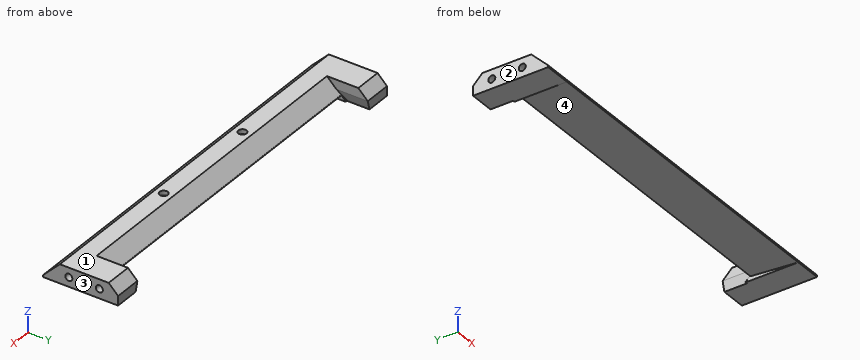
```python
from build123d import *

# Parameters (mm, degrees)
F0_W      = 520.7
F0_H      = 101.6
F1_DEPTH  = 25.4
F2_SIZE   = 22.86
F3_W      = 446.0748
F3_H      = 55.118
F4_DEPTH  = 25.401
F6_DEPTH  = 55.118
F7_SIZE   = 12.7
F9_DEPTH  = 228.6
F10_R     = 5.55625
F11_DEPTH = 6.35
F12_R     = 4.7625
F13_DEPTH = 19.05
F15_DEPTH = 224.028
F16_R     = 0.81661


# Not quite as in the source:
# - a pattern or mirror of a feature is missing from the dataset's text; its kind, count and spacing are read off the source's solid


with BuildPart() as f1:
    # F0 (on Top) → F1 (new body)
    with BuildSketch(Plane.XY):
        with Locations((0, 50.8)):
            Rectangle(F0_W, F0_H)
    extrude(amount=F1_DEPTH)

    # F2
    f2_edges = [f1.edges().sort_by_distance(p)[0] for p in [
        (0, 0, 25.4),
    ]]
    chamfer(f2_edges, length=F2_SIZE)

    # F3 (on face) → F4 (cut, through all)
    with BuildSketch(Plane.XY.offset(25.4)):
        with Locations((0, 74.041)):
            Rectangle(F3_W, F3_H)
    extrude(amount=-F4_DEPTH, mode=Mode.SUBTRACT)

    # F5 (on face) → F6 (cut, through all)
    with BuildSketch(Plane(origin=(0, 101.6, 0), x_dir=(-1, 0, 0), z_dir=(0, 1, 0))):
        Polygon((-223.0374, 0), (-223.0374, 12.7), (-226.4403547439, 0), align=None)
        Polygon((223.0374, 0), (226.4403547439, 0), (223.0374, 12.7), align=None)
    extrude(amount=-F6_DEPTH, mode=Mode.SUBTRACT)

    # F7
    f7_edges = [f1.edges().sort_by_distance(p)[0] for p in [
        (241.6937, 101.6, 25.4),
        (-241.6937, 101.6, 25.4),
    ]]
    chamfer(f7_edges, length=F7_SIZE)

    # F8 (on Right) → F9 (join, symmetric)
    with BuildSketch(Plane.YZ):
        Polygon((71.0692, 0.8128), (46.482, 25.4), (46.482, 0), (71.0692, 0), align=None)
    extrude(amount=F9_DEPTH, both=True)

    # F10 (on face) → F11 (cut)
    with BuildSketch(Plane.XY.offset(25.4)):
        with Locations((76.2, 34.671)):
            Circle(F10_R)
        with Locations((-76.2, 34.671)):
            Circle(F10_R)
    extrude(amount=-F11_DEPTH, mode=Mode.SUBTRACT)

    # F12 (on face) → F13 (cut)
    with BuildSketch(Plane.YZ.offset(260.35)):
        with Locations((34.925, 12.7)):
            Circle(F12_R)
        with Locations((76.2, 12.7)):
            Circle(F12_R)
    f13 = extrude(amount=-F13_DEPTH, mode=Mode.SUBTRACT)

    # F13_copies: F13 across plane
    add(f13.mirror(Plane(origin=(0, 0, 0), x_dir=(0, 0, -1), z_dir=(-1, 0, 0))), mode=Mode.SUBTRACT)

    # F14 (on Right) → F15 (cut, symmetric)
    with BuildSketch(Plane.YZ):
        Polygon((106.9563822457, 9.3574709382), (0, 0), (107.775054872, 0), align=None)
    extrude(amount=F15_DEPTH, both=True, mode=Mode.SUBTRACT)

    # F16
    f16_edges = [f1.edges().sort_by_distance(p)[0] for p in [
        (0, 66.09908, 5.78292),
    ]]
    fillet(f16_edges, radius=F16_R)


solid = f1.part
```
Model file for the job. Use its own axes, mm. Face numbers are marked on the shaded views. Coordinates: 2 decimals unless noted, no trailing zeros. Write each loop counter-clockwise with the first axis right and the second up, starting at its lowest first coordinate (ties: lowest second). Pieces come first, ordered by that corner, then holes. Notation, with made-up numbers: (-36, -31) - (-10, -31) arc R25 ccw to (-10, -16) - close; hole circle Ø10 at (11.25, -19.75). An arc over 180 degrees is marked (long way). Use a Markdown table: item, result. Add a question column.
Item 1: Band-saw the part on A-A, the plane y = 76.2. Write the cut outline in (x, z), and give its area (3 significant figures).
Item 2: Two-plate mould, pull along X, no slides. Class the marked faces 1, 2, 3 and 4: pulls with the +X half, pulls with the -X half, needs draft (parallel to the pull), parting line crosses it, or undercut.
Item 3: Band-saw the part on D-D, the plane y = 15. Write the cut outline in (x, z), and give its area (3 significant figures).
Item 4: Band-saw the part on C-C, the plane x = -76.2. Write the cut outline in (y, z).
Item 5: Band-saw the part on B-B, the plane y = 52.5. Write the cut outline in (x, z).
Item 6: Drop flat-ended pins along their axis: pin 1 (5 mm diameter, centred on x = 36, z = 14, fed in from -Y); pin 2 (1.5 mm diameter, centred on x = 59.5, y = 31, fed in from -Z); pin 3 (0.7 mm diameter, centred on x = -225, z = 0.5, fed in from +Y). Give the stop position or say it passes through.
Item 7: Drill centre lines: line 1 along Z through (x, y) = (250.5, 76.2); line 2 along X through (y, z) = (87, 16.75); line 3 along X through (y, z) = (31, 23.75). Where is each one in solid material? Low to high.
A:
| question | item | result |
|---|---|---|
| 1 | outline | (-260.35, 0) - (-226.44, 0) - (-223.04, 12.7) - (-223.04, 25.4) - (-260.35, 25.4) - (-260.35, 17.46) - (-241.3, 17.46) - (-241.3, 7.94) - (-260.35, 7.94) - close; (223.04, 12.7) - (226.44, 0) - (260.35, 0) - (260.35, 7.94) - (241.3, 7.94) - (241.3, 17.46) - (260.35, 17.46) - (260.35, 25.4) - (223.04, 25.4) - close |
| 1 | area | 1,490 mm² |
| 2 | face 1 | needs draft |
| 2 | face 2 | pulls with the -X half |
| 2 | face 3 | pulls with the +X half |
| 2 | face 4 | undercut |
| 3 | outline | (-260.35, 0) - (-224.03, 0) - (-224.03, 1.31) - (224.03, 1.31) - (224.03, 0) - (260.35, 0) - (260.35, 17.54) - (-260.35, 17.54) - close |
| 3 | area | 8,550 mm² |
| 4 | outline | (0, 0) - (64.35, 5.63) arc R0.82 ccw to (64.86, 7.02) - (46.48, 25.4) - (40.23, 25.4) - (40.23, 19.05) - (29.11, 19.05) - (29.11, 25.4) - (22.86, 25.4) - (0, 2.54) - close |
| 5 | outline | (-260.35, 0) - (-224.03, 0) - (-224.03, 4.59) - (224.03, 4.59) - (224.03, 0) - (260.35, 0) - (260.35, 25.4) - (223.04, 25.4) - (223.04, 19.38) - (-223.04, 19.38) - (-223.04, 25.4) - (-260.35, 25.4) - close |
| 6 | pin 1 | stops at y = 8.96 |
| 6 | pin 2 | stops at z = 2.65 |
| 6 | pin 3 | stops at y = 71.07 |
| 7 | line 1 | z = 0 to 7.94, 17.46 to 25.4 |
| 7 | line 2 | x = -260.35 to -223.04, 223.04 to 260.35 |
| 7 | line 3 | x = -260.35 to -80.37, -72.03 to 72.03, 80.37 to 260.35 |
